```python
from build123d import *

# Parameters (mm, degrees)
BOSS_EXTRUDE1_START = -3.775
SKETCH1_W           = 16.2
SKETCH1_H           = 32.8
BOSS_EXTRUDE1_DEPTH = 10.275
BOSS_EXTRUDE2_START = -65.25
SKETCH2_W           = 13
SKETCH2_H           = 11.7
BOSS_EXTRUDE2_DEPTH = 2.25
BOSS_EXTRUDE3_START = 82.6
SKETCH3_R           = 6.5
BOSS_EXTRUDE3_DEPTH = 2.1
BOSS_EXTRUDE4_START = 82.6
SKETCH4_W           = 19
SKETCH4_H           = 13
BOSS_EXTRUDE4_DEPTH = 2.1
CUT_EXTRUDE1_START  = 82.6
SKETCH5_R           = 3.55
CUT_EXTRUDE1_DEPTH  = 2.1
CUT_EXTRUDE2_START  = 82.6
CUT_EXTRUDE2_DEPTH  = 2.1
BOSS_EXTRUDE5_START = 44
SKETCH7_R           = 6.5
BOSS_EXTRUDE5_DEPTH = 1.5
BOSS_EXTRUDE6_START = 44
SKETCH8_W           = 19
SKETCH8_H           = 13
BOSS_EXTRUDE6_DEPTH = 1.5
CUT_EXTRUDE3_START  = 44
SKETCH9_R           = 2.95
CUT_EXTRUDE3_DEPTH  = 1.5
CUT_EXTRUDE4_START  = -2.125
SKETCH10_W          = 13
SKETCH10_H          = 23.2
CUT_EXTRUDE4_DEPTH  = 8.625
CUT_EXTRUDE5_START  = 3.5
SKETCH11_R          = 1
CUT_EXTRUDE5_DEPTH  = 3
CUT_EXTRUDE6_START  = 3.5
SKETCH12_R          = 1
CUT_EXTRUDE6_DEPTH  = 3
CUT_EXTRUDE7_START  = -12.75
SKETCH13_R          = 3.15
CUT_EXTRUDE7_DEPTH  = 1.3
CUT_EXTRUDE8_START  = 73
SKETCH14_W          = 4.4
SKETCH14_H          = 6
CUT_EXTRUDE8_DEPTH  = 2.4


with BuildPart() as part:
    # Sketch1 → Boss-Extrude1 (new, symmetric)
    with BuildSketch(Plane.XY.offset(BOSS_EXTRUDE1_START)):
        with Locations((-59.4, 59)):
            Rectangle(SKETCH1_W, SKETCH1_H)
    extrude(amount=BOSS_EXTRUDE1_DEPTH, both=True)

    # Sketch2 → Boss-Extrude2 (add, symmetric)
    with BuildSketch(Plane(origin=(0, 0, 0), x_dir=(0, 0, -1), z_dir=(1, 0, 0)).offset(BOSS_EXTRUDE2_START)):
        with Locations((0, 78.85)):
            Rectangle(SKETCH2_W, SKETCH2_H)
    extrude(amount=BOSS_EXTRUDE2_DEPTH, both=True)



with BuildPart() as body_2:
    # Sketch3 → Boss-Extrude3 (new, symmetric)
    with BuildSketch(Plane(origin=(0, 0, 0), x_dir=(1, 0, 0), z_dir=(0, 1, 0)).offset(BOSS_EXTRUDE3_START)):
        with Locations(Location((-85, 0, 0), (0, 0, 270))):
            Circle(SKETCH3_R)
    extrude(amount=BOSS_EXTRUDE3_DEPTH, both=True)


with BuildPart() as part_1:
    add(part.part)

    add(body_2.part)  # Boss-Extrude4 merges body 2
    # Sketch4 → Boss-Extrude4 (add, symmetric)
    with BuildSketch(Plane(origin=(0, 0, 0), x_dir=(1, 0, 0), z_dir=(0, 1, 0)).offset(BOSS_EXTRUDE4_START)):
        with Locations((-75.5, 0)):
            Rectangle(SKETCH4_W, SKETCH4_H)
    extrude(amount=BOSS_EXTRUDE4_DEPTH, both=True)

    # Sketch5 → Cut-Extrude1 (cut, symmetric)
    with BuildSketch(Plane(origin=(0, 0, 0), x_dir=(1, 0, 0), z_dir=(0, 1, 0)).offset(CUT_EXTRUDE1_START)):
        with Locations(Location((-85, 0, 0), (0, 0, 270))):
            Circle(SKETCH5_R)
    extrude(amount=CUT_EXTRUDE1_DEPTH, both=True, mode=Mode.SUBTRACT)

    # Sketch6 → Cut-Extrude2 (cut, symmetric)
    with BuildSketch(Plane(origin=(0, 0, 0), x_dir=(1, 0, 0), z_dir=(0, 1, 0)).offset(CUT_EXTRUDE2_START)):
        Polygon((-85, -3.55), (-72.3, -2.403281405), (-72.3, 2.403281405), (-85, 3.55), align=None)
    extrude(amount=CUT_EXTRUDE2_DEPTH, both=True, mode=Mode.SUBTRACT)



with BuildPart() as body_2_2:
    # Sketch7 → Boss-Extrude5 (new, symmetric)
    with BuildSketch(Plane(origin=(0, 0, 0), x_dir=(1, 0, 0), z_dir=(0, 1, 0)).offset(BOSS_EXTRUDE5_START)):
        with Locations(Location((-85, 0, 0), (0, 0, 270))):
            Circle(SKETCH7_R)
    extrude(amount=BOSS_EXTRUDE5_DEPTH, both=True)


with BuildPart() as part_2:
    add(part_1.part)

    add(body_2_2.part)  # Boss-Extrude6 merges body 2 2
    # Sketch8 → Boss-Extrude6 (add, symmetric)
    with BuildSketch(Plane(origin=(0, 0, 0), x_dir=(1, 0, 0), z_dir=(0, 1, 0)).offset(BOSS_EXTRUDE6_START)):
        with Locations((-75.5, 0)):
            Rectangle(SKETCH8_W, SKETCH8_H)
    extrude(amount=BOSS_EXTRUDE6_DEPTH, both=True)

    # Sketch9 → Cut-Extrude3 (cut, symmetric)
    with BuildSketch(Plane(origin=(0, 0, 0), x_dir=(1, 0, 0), z_dir=(0, 1, 0)).offset(CUT_EXTRUDE3_START)):
        with Locations(Location((-85, 0, 0), (0, 0, 270))):
            Circle(SKETCH9_R)
    extrude(amount=CUT_EXTRUDE3_DEPTH, both=True, mode=Mode.SUBTRACT)

    # Sketch10 → Cut-Extrude4 (cut, symmetric)
    with BuildSketch(Plane.XY.offset(CUT_EXTRUDE4_START)):
        with Locations((-59.4, 59)):
            Rectangle(SKETCH10_W, SKETCH10_H)
    extrude(amount=CUT_EXTRUDE4_DEPTH, both=True, mode=Mode.SUBTRACT)

    # Sketch11 → Cut-Extrude5 (cut, symmetric)
    with BuildSketch(Plane.XY.offset(CUT_EXTRUDE5_START)):
        with Locations((-59.4, 45.25)):
            Circle(SKETCH11_R)
    extrude(amount=CUT_EXTRUDE5_DEPTH, both=True, mode=Mode.SUBTRACT)

    # Sketch12 → Cut-Extrude6 (cut, symmetric)
    with BuildSketch(Plane.XY.offset(CUT_EXTRUDE6_START)):
        with Locations((-59.4, 72.75)):
            Circle(SKETCH12_R)
    extrude(amount=CUT_EXTRUDE6_DEPTH, both=True, mode=Mode.SUBTRACT)

    # Sketch13 → Cut-Extrude7 (cut, symmetric)
    with BuildSketch(Plane.XY.offset(CUT_EXTRUDE7_START)):
        with Locations((-59.4, 64.5)):
            Circle(SKETCH13_R)
    extrude(amount=CUT_EXTRUDE7_DEPTH, both=True, mode=Mode.SUBTRACT)

    # Sketch14 → Cut-Extrude8 (cut, symmetric)
    with BuildSketch(Plane(origin=(0, 0, 0), x_dir=(1, 0, 0), z_dir=(0, 1, 0)).offset(CUT_EXTRUDE8_START)):
        with Locations((-59.4, 7.75)):
            Rectangle(SKETCH14_W, SKETCH14_H)
    extrude(amount=CUT_EXTRUDE8_DEPTH, both=True, mode=Mode.SUBTRACT)


solid = part_2.part
```
Geometry check sheet. Reference: the model listing, model coordinates, mm. A direction names the side the tool comes from. Round coordinates to 2 decimals unless told otherwise and drop trailing zeros. Order: outer loops, then holes, each group sorted by start corner. A loop starts at its lowest first (then second) coordinate and runs counter-clockwise, first axis right, second up. Notation, with made-up numbers: (46, 36) - (56, 36) arc R24 cw to (56, 66) - close; hole circle Ø5 at (27.5, 46.25). An arc over 180 degrees is marked (long way). Use a Markdown table: item, result. Add a question column.
1) Mould release check, pull along X, two halves, no side actions. Record for faces 4 (the flat face through (-59, 70.6, -2)), 5 (the cylindrical face through (-91.5, 82.6, -0.1)), 6 (the cylindrical face through (-58.476, 72.367, 3.542)), 7 (the flat face through (-74, 84.7, -3)): released by +X, released by -X, zero draft, split by the parting line, or undercut.
2) Set-up check for faces 1 (the flat face through (-57.2, 73, -8)), 2 (the flat face through (-77, 80.5, -3)), 3 (the flat face through (-59, 47.4, -2)): record each of +Z, -Z, +X, -X, +Y, -Y from which the full face is reachable in a straight line by a thin tool's end or side.
3) Section check A-A (z = 0). Record the cut outline in (x, y).
4) Section check B-B (x = -59.4). Record the cut outline in (y, z), then the cut area to 3 significant figures.
5) Section check D-D (x = -85.5). Record the cut outline in (y, z), then the cut area to 3 significant figures.
6) Section check C-C (y = 72.75). Record the cut outline in (x, z).
7) Thickness scan on line 1 along Y through (x, z) = (-59.4, 4.9); line 2 along X through (y, z) = (72.75, 1.9); line 3 along X through (y, z) = (74, -8.25). Record the ranges inside material, lowest first.
8) Gauge pin test, flat ends, axial feed: P1, Ø4, axis at x = -60, z = -1.5, coming from the +Y side; P2, Ø4, axis at x = -57.5, z = -4.5, coming from the -Y side; P3, Ø6, axis at x = -78, y = 75, coming from the -Z side; P4, Ø12, axis at y = 54, z = 3.5, coming from the -X side. Record the tip position at first contact, or that the pin passes through.
Established:
| question | item | result |
|---|---|---|
| 1 | face 4 | undercut |
| 1 | face 5 | released by -X |
| 1 | face 6 | undercut |
| 1 | face 7 | zero draft |
| 2 | face 1 | +Y |
| 2 | face 2 | +Z, -Z, -X |
| 2 | face 3 | +Z |
| 3 | outline | (-91.5, 42.5) - (-87.95, 42.5) - (-87.95, 45.5) - (-91.5, 45.5) - close; (-91.5, 80.5) - (-88.55, 80.5) - (-88.55, 84.7) - (-91.5, 84.7) - close; (-82.05, 42.5) - (-66, 42.5) - (-66, 42.6) - (-51.3, 42.6) - (-51.3, 75.4) - (-63, 75.4) - (-63, 84.7) - (-72.3, 84.7) - (-72.3, 80.5) - (-67.5, 80.5) - (-67.5, 45.5) - (-82.05, 45.5) - close; hole (-65.9, 47.4) - (-52.9, 47.4) - (-52.9, 70.6) - (-65.9, 70.6) - close |
| 4 | outline | (42.6, -14.05) - (61.35, -14.05) - (61.35, -11.45) - (67.65, -11.45) - (67.65, -14.05) - (75.4, -14.05) - (75.4, -10.75) - (47.4, -10.75) - (47.4, 6.5) - (46.25, 6.5) - (46.25, 0.5) - (44.25, 0.5) - (44.25, 6.5) - (42.6, 6.5) - close; (70.6, -4.75) - (75.4, -4.75) - (75.4, 6.5) - (73.75, 6.5) - (73.75, 0.5) - (71.75, 0.5) - (71.75, 6.5) - (70.6, 6.5) - close |
| 4 | area | 205 mm2 |
| 5 | outline | (42.5, -6.48) - (45.5, -6.48) - (45.5, -2.91) - (42.5, -2.91) - close; (42.5, 2.91) - (45.5, 2.91) - (45.5, 6.48) - (42.5, 6.48) - close; (80.5, -6.48) - (84.7, -6.48) - (84.7, -3.51) - (80.5, -3.51) - close; (80.5, 3.51) - (84.7, 3.51) - (84.7, 6.48) - (80.5, 6.48) - close |
| 5 | area | 46.4 mm2 |
| 6 | outline | (-67.5, -14.05) - (-51.3, -14.05) - (-51.3, 6.5) - (-58.4, 6.5) - (-58.4, 0.5) - (-60.4, 0.5) - (-60.4, 6.5) - (-67.5, 6.5) - close; hole (-61.6, -10.75) - (-57.2, -10.75) - (-57.2, -4.75) - (-61.6, -4.75) - close |
| 7 | line 1 | 42.6 to 44.25, 46.25 to 47.4, 70.6 to 71.75, 73.75 to 75.4 |
| 7 | line 2 | -67.5 to -60.4, -58.4 to -51.3 |
| 7 | line 3 | -67.5 to -61.6, -57.2 to -51.3 |
| 8 | P1 | y = 75.4 |
| 8 | P2 | y = 42.6 |
| 8 | P3 | through |
| 8 | P4 | x = -67.5 |
